Part model, mm, in its own coordinate system. A direction names the side the tool comes from. Round coordinates to 2 decimals unless told otherwise and drop trailing zeros. Write each loop counter-clockwise with the first axis right and the second up, starting at its lowest first coordinate (ties: lowest second). Pieces come first, ordered by that corner, then holes.
Autodesk Inventor part; units mm, degrees
ref_plane "YZ Plane" through (0, 0, 0) normal (1, 0, 0) x (0, 1, 0)
ref_plane "XZ Plane" through (0, 0, 0) normal (0, 1, 0) x (-1, 0, 0)
ref_plane "XY Plane" through (0, 0, 0) normal (0, 0, 1) x (1, 0, 0)
sketch "Sketch1" plane through (0, 0, 0) normal (0, 1, 0) x (-1, 0, 0)
  line L0 (0, 0) -> (0, -63.5)
  line L1 (0, -63.5) -> (3.175, -63.5)
  line L2 (3.175, -63.5) -> (3.175, 0)
  line L3 (3.175, 0) -> (0, 0)
  line L4 (3.175, 0) -> (15.875, 0)
  line L5 (15.875, 0) -> (69.7565, -53.8815)
  line L6 (69.7565, -53.8815) -> (69.7565, -66.5815)
  line L7 (69.7565, -66.5815) -> (69.7565, -69.7565)
  line L8 (69.7565, -69.7565) -> (6.2565, -69.7565)
  line L9 (6.2565, -69.7565) -> (6.2565, -66.5815)
  line L10 (6.2565, -66.5815) -> (69.7565, -66.5815)
  arc A0 (6.2565, -66.5815) -> (3.175, -63.5) centre (4.7158, -65.0408) ccw
  circle A1 centre (10.1629, -59.5936) radius 3.6195
  line L11 (10.1629, -55.9741) -> (10.1629, -43.8456) construction
  circle A2 centre (10.1629, -41.8136) radius 2.032
  line L12 (13.7824, -59.5936) -> (25.9236, -59.5936) construction
  circle A3 centre (27.9556, -59.5936) radius 2.032
  line L13 (6.2565, -63.5) -> (42.8158, -26.9408) construction
  circle A4 centre (27.6295, -42.127) radius 14.224
  circle A5 centre (46.1715, -42.127) radius 2.032
  line L14 (27.6295, -27.903) -> (27.6295, -25.617) construction
  circle A6 centre (27.6295, -23.585) radius 2.032
  circle A7 centre (47.0691, -59.5936) radius 3.7465
  line L15 (10.1629, -39.7816) -> (10.1629, -26.4466) construction
  circle A8 centre (10.1629, -22.7001) radius 3.7465
  dimension "d6" = 63.5
  dimension "d7" = 3.175
  dimension "d8" = 12.7
  dimension "d9" = 76.2
  dimension "d10" = 135
  dimension "d11" = 12.7
  dimension "d12" = 3.175
  dimension "d13" = 63.5
  dimension "d14" = 3.175
  dimension "d18" = 12.1285
  dimension "d20" = 12.1412
  dimension "d26" = 2.286
  dimension "d30" = 13.335
extrude "Extrusion1" add sketch "Sketch1" along normal blind 3.175 contours L4 L5 L6 L10 A0 L2
extrude "Extrusion2" add sketch "Sketch1" along normal blind 25.4 contours L3 L2 L1 L0 | L10 L7 L8 L9
chamfer "Chamfer1" distance 3.175 angle 45 4 edges at (-6.2565, 25.4, -68.169) (-1.5875, 25.4, -63.5) (-1.5875, 25.4, 0) (-69.7565, 25.4, -68.169)
sketch "Sketch2" plane through (0, 0, 0) normal (1, 0, 0) x (0, 0, -1)
  line L0 (0, 3.175) -> (0, 22.225)
  circle A0 centre (6.35, 12.7) radius 1.5875
  circle A1 centre (19.05, 12.7) radius 1.5875
  circle A2 centre (31.75, 12.7) radius 1.5875
  circle A3 centre (44.45, 12.7) radius 1.5875
  circle A4 centre (57.15, 12.7) radius 1.5875
  point P0 (0, 0)
  dimension "d44" = 3.175
  dimension "d46" = 3.175
  dimension "d48" = 3.175
  dimension "d50" = 3.175
sketch "Sketch3" plane through (-6.2565, 0, -69.7565) normal (0, 0, -1) x (-1, 0, 0)
  line L0 (0, 0) -> (0, 22.225)
  circle A0 centre (6.35, 11.1125) radius 1.5875
  circle A1 centre (19.05, 11.1125) radius 1.5875
  circle A2 centre (31.75, 11.1125) radius 1.5875
  circle A3 centre (44.45, 11.1125) radius 1.5875
  circle A4 centre (57.15, 11.1125) radius 1.5875
  point P0 (-6.2565, 0)
  dimension "d54" = 3.175
  dimension "d56" = 3.175
  dimension "d58" = 3.175
  dimension "d60" = 3.175
  dimension "d62" = 3.175
extrude "Extrusion3" cut sketch "Sketch2" against normal blind 3.175
extrude "Extrusion4" cut sketch "Sketch3" against normal blind 3.175
fillet "Fillet1" radius 3.175 2 edges at (0, 0, -31.75) (-38.0065, 0, -69.7565)
properties part number "triangular L-bracket"
Q1. Saw through at B-B, the plane z = -48. Write the cut outline in (x, y) (3 decimals), and give its area (3 significant figures).
Q2. Two-plate mould, pull along Y, no slides. Class faces 1 (the cylindrical face through (-16.342, 1.565, -33.472)), 2 (the cylindrical face through (-37.8, 12.686, -68.191)), 3 (the cylindrical face through (-23.72, 11.18, -68.19)), 4 (the flat face through (-43, 0, -40)): released by +Y, released by -Y, zero draft, split by the parting line, or undercut.
Q3. Saw through at A-A, the plane y = 6.25. Write the cut outline in (x, z) (1 decimal).
Q4. Wall check: line 1 (Y direction, x = -52.5, z = -66) (3 decimals); line 2 (Z direction, x = -58.5, y = 12.25); line 3 (X direction, y = 12.75, z = -55) (3 decimals). Give the ranges that are in metal, low to high.
Q5. Tool access for faces 5 (the cylindrical face through (-0.91, 0.95, -32.19)), 6 (the flat face through (-3.175, 17, -32)): list every direction of +Z, -Z, +X, -X, +Y, -Y with a clear straight run to the whole face (end or side of a thin tool).
Q6. Saw through at C-C, the plane z = -31.5. Write the cut outline in (x, y) (3 decimals).
Q7. Drop flat-ended pins along their axis: P1, Ø2.5, axis at x = -63.41, y = 11.11, coming from the -Z side; P2, Ø3.5, axis at x = -25.31, y = 11.11, coming from the +Z side; P3, Ø1.6, axis at y = 13, z = -68.5, coming from the +X side; P4, Ø10, axis at x = -14.5, z = -61.5, coming from the +Y side (3 decimals). Give the stop position or say it passes through.
Computed:
1. outline: (-63.875, 0) - (-40.584, 0) - (-40.584, 3.175) - (-63.875, 3.175) - close; (-14.675, 0) - (-3.175, 0) arc R3.175 ccw to (0, 3.175) - (0, 25.4) - (-3.175, 25.4) - (-3.175, 3.175) - (-14.675, 3.175) - close
1. area: 189 mm2
2. face 1: zero draft
2. face 2: undercut
2. face 3: undercut
2. face 4: released by -Y
3. outline: (-69.8, -69.8) - (-6.3, -69.8) - (-6.3, -66.6) - (-69.8, -66.6) - close; (-3.2, -63.5) - (0, -63.5) - (0, 0) - (-3.2, 0) - close
4. line 1: y = 0 to 3.175
4. line 2: z = -69.76 to -66.58
4. line 3: x = -3.175 to 0
5. face 5: +Z, -Z, +X, -Y
5. face 6: +Z, -Z, -X, +Y
6. outline: (-47.375, 0) - (-37.084, 0) - (-37.084, 3.175) - (-47.375, 3.175) - close; (-18.175, 0) - (-3.175, 0) arc R3.175 ccw to (0, 3.175) - (0, 11.132) - (-3.175, 11.132) - (-3.175, 3.175) - (-18.175, 3.175) - close; (-3.175, 14.268) - (0, 14.268) - (0, 25.4) - (-3.175, 25.4) - close
7. P1: passes through
7. P2: stops at z = -66.58
7. P3: stops at x = -6.26
7. P4: stops at y = 3.175
